The listing builds one solid part. Answer for the finished solid, in the listing's coordinates (mm). Round coordinates to 2 decimals unless told otherwise and drop trailing zeros. Order: outer loops, then holes, each group sorted by start corner. A loop starts at its lowest first (then second) coordinate and runs counter-clockwise, first axis right, second up. Notation, with made-up numbers: M 43.25,-38.75 L 98.25,-38.75 A30 ccw 98.25,-7.75 Z; hole C 30.25,39.25 d11. An arc over 180 degrees is marked long. Put each result on its own line as item: value. Start each with the question number.
1. The part is cut by section A-A (y = 3.5). Give the vertices of the cut face in (x, z).
2. Each of these flat-tipped pins is pushed along its axis until it touches: pin 1 Ø1 at (x, y) = (88, 2.5) entering from +Z; pin 2 Ø5 at (x, z) = (-118.5, 18) entering from +Y; pin 3 Ø1.5 at (x, z) = (-118.5, 18.5) entering from -Y; pin 4 Ø4 at (x, y) = (-88.5, 4.5) entering from -Z. Where does it stop, or does it pass through?
3. The part is cut by section D-D (z = -8.5). Give the vertices of the cut face in (x, y).
4. The part is cut by section C-C (x = -22.5). Give the vertices of the cut face in (y, z).
5. The part is cut by section B-B (x = -130). Give the vertices of the cut face in (y, z), then the cut area to 3 significant figures.
6. Consider line 1 (Z direction, x = 111.5, y = 9.75); line 2 (Z direction, x = -130, y = 7); line 3 (X direction, y = 9, z = -4). Determine where each line is inside the solid, lowest interval first.
from build123d import *

# Parameters (mm, degrees)
BOSS_EXTRU_1_DEPTH      = 10
SYM_TRIE8_COPY_1_DEPTH  = 10
ESQUISSE2_R             = 3.5
ESQUISSE2_R_2           = 6
ESQUISSE2_R_3           = 3.25
ENL_V_MAT_EXTRU_1_DEPTH = 10


with BuildPart() as part:
    # Esquisse1 → Boss.-Extru.1 (new body)
    with BuildSketch(Plane(origin=(0, 0, 0), x_dir=(1, 0, 0), z_dir=(0, 1, 0))):
        with BuildLine():
            Line((-30.324962458, 26.084413966), (-136.567926949, 14.917828431))
            ThreePointArc((-136.567926949, 14.917828431), (-146.147172382, 10.036959095), (-150, 0))
            Line((-150, 0), (0, 0))
            Line((0, 0), (0, 40))
            ThreePointArc((0, 40), (-16.682677264, 36.355031004), (-30.324962458, 26.084413966))
        make_face()
    boss_extru_1 = extrude(amount=BOSS_EXTRU_1_DEPTH)

    # Symétrie1: Boss.-Extru.1 across plane
    add(boss_extru_1.mirror(Plane(origin=(-150, 10, 0), x_dir=(1, 0, 0), z_dir=(0, 0, -1))))

    # Symétrie8: Boss.-Extru.1 across plane
    add(boss_extru_1.mirror(Plane(origin=(0, 0, 0), x_dir=(0, 0, 1), z_dir=(1, 0, 0))))

    # Symétrie8 copy 1 sketch → Symétrie8 copy 1 (add)
    with BuildSketch(Plane(origin=(0, 0, 0), x_dir=(-1, 0, 0), z_dir=(0, 1, 0))):
        with BuildLine():
            Line((-30.324962458, 26.084413966), (-136.567926949, 14.917828431))
            ThreePointArc((-136.567926949, 14.917828431), (-146.147172382, 10.036959095), (-150, 0))
            Line((-150, 0), (0, 0))
            Line((0, 0), (0, 40))
            ThreePointArc((0, 40), (-16.682677264, 36.355031004), (-30.324962458, 26.084413966))
        make_face()
    extrude(amount=SYM_TRIE8_COPY_1_DEPTH)

    # Esquisse2 → Enlèv. mat.-Extru.1 (cut)
    with BuildSketch(Plane(origin=(0, 10, 0), x_dir=(1, 0, 0), z_dir=(0, 1, 0))):
        with Locations(Location((-22.5, 0, 0), (0, 0, 270))):
            Circle(ESQUISSE2_R)
        with Locations(Location((22.5, 0, 0), (0, 0, 270))):
            Circle(ESQUISSE2_R)
        with Locations(Location((0, 0, 0), (0, 0, 270))):
            Circle(ESQUISSE2_R_2)
        with Locations(Location((-110, 0, 0), (0, 0, 270))):
            Circle(ESQUISSE2_R_3)
        with Locations(Location((-130, 0, 0), (0, 0, 270))):
            Circle(ESQUISSE2_R_3)
        with Locations(Location((110, 0, 0), (0, 0, 270))):
            Circle(ESQUISSE2_R_3)
        with Locations(Location((130, 0, 0), (0, 0, 270))):
            Circle(ESQUISSE2_R_3)
    extrude(amount=-ENL_V_MAT_EXTRU_1_DEPTH, mode=Mode.SUBTRACT)


solid = part.part
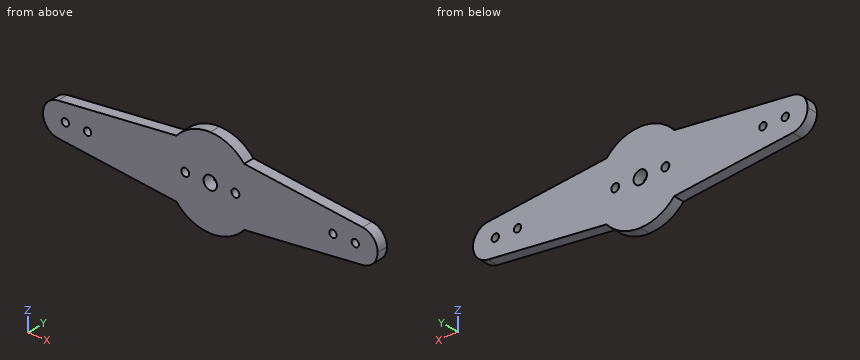
Resolved:
1. outline: M -136.57,-14.92 L -30.32,-26.08 A40 ccw 30.32,-26.08 L 136.57,-14.92 A15 ccw 136.57,14.92 L 30.32,26.08 A40 ccw -30.32,26.08 L -136.57,14.92 A15 ccw Z; hole C -130,0 d6.5; hole C -110,0 d6.5; hole C -22.5,0 d7; hole C 0,0 d12; hole C 22.5,0 d7; hole C 110,0 d6.5; hole C 130,0 d6.5
2. pin 1: z = 20.08
2. pin 2: y = 10
2. pin 3: through
2. pin 4: z = -20.18
3. outline: M -147.36,0 L 147.36,0 L 147.36,10 L -147.36,10 Z
4. outline: M 0,-33.07 L 10,-33.07 L 10,-3.5 L 0,-3.5 Z; M 0,3.5 L 10,3.5 L 10,33.07 L 0,33.07 Z
5. outline: M 0,-15.61 L 10,-15.61 L 10,-3.25 L 0,-3.25 Z; M 0,3.25 L 10,3.25 L 10,15.61 L 0,15.61 Z
5. area: 247 mm2
6. line 1: -17.55 to -2.88, 2.88 to 17.55
6. line 2: -15.61 to -3.25, 3.25 to 15.61
6. line 3: -149.46 to -4.47, 4.47 to 149.46
